Verification items for the finished model (mm, model axes). A direction names the side the tool comes from. Round coordinates to 2 decimals unless told otherwise and drop trailing zeros. Loops run counter-clockwise (first coordinate to the right, second up) from the corner with the lowest first, then second, coordinate; pieces in that order, holes last. Notation, with made-up numbers: M 32,86 L 73,86 A31 cw 73,122 Z; hole C 75,-25.75 d2. An arc over 180 degrees is marked long. Write item = value, one per line. Start each with the question number.
Autodesk Fusion 360 part; units mm, degrees
sketch "Sketch1" plane through (0, 0, 0) normal (0, 1, 0) x (1, 0, 0)
  line L0 (28.15, 28.15) -> (-28.15, 28.15)
  line L1 (-28.15, 28.15) -> (-28.15, -28.15)
  line L2 (-28.15, -28.15) -> (28.15, -28.15)
  line L3 (28.15, -28.15) -> (28.15, 28.15)
  line L4 (28.15, 28.15) -> (-28.15, -28.15) construction
  line L5 (-28.15, 28.15) -> (28.15, -28.15) construction
  line L6 (28.15, 28.15) -> (23.85, 28.15)
  line L7 (23.85, 28.15) -> (23.85, 23.85)
  circle A0 centre (23.85, 23.85) radius 2.5
  circle A1 centre (-23.85, 23.85) radius 2.5
  circle A2 centre (-23.85, -23.85) radius 2.5
  circle A3 centre (23.85, -23.85) radius 2.5
  line L8 (32, 32) -> (-32, 32)
  line L9 (-32, 32) -> (-32, -32)
  line L10 (-32, -32) -> (32, -32)
  line L11 (32, -32) -> (32, 32)
  line L12 (32, 32) -> (-32, -32) construction
  line L13 (-32, 32) -> (32, -32) construction
  circle A4 centre (0, 0) radius 19.25
  dimension "d1" = 56.3
  dimension "d2" = 56.3
  dimension "d3" = 4.3
  dimension "d4" = 4.3
  dimension "d5" = 5
  dimension "d7" = 360
  dimension "d8" = 64
  dimension "d9" = 38.5
extrude "Extrude1" add sketch "Sketch1" along normal blind 4 contours L0 L1 L2 L3 L6 | L8 L9 L10 L11
sketch "Sketch2" plane through (0, 0, 0) normal (0, 1, 0) x (1, 0, 0)
  circle A0 centre (-23.85, 23.85) radius 2.5
  circle A1 centre (23.85, 23.85) radius 2.5
  circle A2 centre (0, 0) radius 19.25
  circle A3 centre (23.85, -23.85) radius 2.5
  circle A4 centre (-23.85, -23.85) radius 2.5
  line L0 (32, 32) -> (32, -32)
  line L1 (32, -32) -> (-32, -32)
  line L2 (-32, -32) -> (-32, 32)
  line L3 (-32, 32) -> (32, 32)
  line L4 (-28.15, 28.15) -> (-28.15, -28.15)
  line L5 (-32, 32) -> (-32, -32)
  line L6 (-28.15, -28.15) -> (-32, -28.15)
  line L7 (-28.15, 28.15) -> (-32, 28.15)
extrude "Extrude2" add sketch "Sketch2" against normal blind 54.2 contours L2 L4 L5 L6 L7
sketch "Sketch3" plane through (-32, 0, 0) normal (-1, 0, 0) x (0, 0, 1)
  line L0 (-32, 0) -> (-28.15, 0)
  line L1 (-28.15, 0) -> (-28.15, -54.2)
  line L2 (-28.15, -54.2) -> (28.15, -54.2)
  line L3 (28.15, -54.2) -> (28.15, 0)
  line L4 (28.15, 0) -> (32, 0)
  line L5 (32, 0) -> (32, 4)
  line L6 (32, 4) -> (-32, 4)
  line L7 (-32, 4) -> (-32, 0)
  line L8 (0, -54.2) -> (10, -54.2)
  line L9 (10, -54.2) -> (-10, -54.2)
  line L10 (-10, -54.2) -> (-10, -49.2)
  line L11 (-10, -49.2) -> (10, -49.2)
  line L12 (10, -49.2) -> (10, -54.2)
  dimension "d14" = 10
  dimension "d15" = 20
  dimension "d16" = 5
extrude "Extrude3" add sketch "Sketch3" along normal blind 15 contours L2 L8 L9 L10 L11 L12
sketch "Sketch4" plane through (0, -49.2, 0) normal (0, 1, 0) x (-1, 0, 0)
  line L0 (32, 10) -> (32, -10)
  line L1 (32, -10) -> (47, -10)
  line L2 (47, -10) -> (47, 10)
  line L3 (47, 10) -> (32, 10)
  line L4 (32, 0) -> (39, 0)
  circle A0 centre (39, 0) radius 2.75
  dimension "d19" = 7
  dimension "d20" = 5.5
extrude "Extrude4" cut sketch "Sketch4" against normal blind 19 contours A0
extrude "Extrude7" cut sketch "Sketch1" along normal blind 5 contours L8 L9 L10 L11
sketch "Sketch7" plane through (0, 0, 0) normal (0, 1, 0) x (1, 0, 0)
  line L0 (-28.15, 28.15) -> (-28.15, -28.15)
  line L1 (-28.15, -28.15) -> (28.15, -28.15)
  line L2 (28.15, -28.15) -> (28.15, 28.15)
  line L3 (28.15, 28.15) -> (-28.15, 28.15)
  circle A0 centre (-23.85, 23.85) radius 2.5
  circle A1 centre (23.85, 23.85) radius 2.5
  circle A2 centre (0, 0) radius 19.25
  circle A3 centre (23.85, -23.85) radius 2.5
  circle A4 centre (-23.85, -23.85) radius 2.5
  line L4 (-28.15, -28.15) -> (-32, -28.15)
  line L5 (-28.15, 28.15) -> (-32, 28.15)
  line L6 (-32, 28.15) -> (-32, -28.15)
  line L7 (-28.15, -28.15) -> (-28.15, 28.15)
extrude "Extrude8" add sketch "Sketch7" along normal blind 4 contours L0 L4 L5 L6 L7
sketch "Sketch8" plane through (-28.15, 0, 0) normal (1, 0, 0) x (0, 0, -1)
  line L0 (28.15, 0) -> (-28.15, 0)
  line L1 (-28.15, 0) -> (-28.15, -54.2)
  line L2 (-28.15, -54.2) -> (28.15, -54.2)
  line L3 (28.15, -54.2) -> (28.15, 0)
  line L4 (-28.15, -54.2) -> (-18.15, -54.2)
  line L5 (-18.15, -54.2) -> (-28.15, -54.2)
  line L6 (-28.15, -54.2) -> (-28.15, 0)
  line L7 (-28.15, 0) -> (-18.15, 0)
  line L8 (-18.15, 0) -> (-18.15, -54.2)
  line L9 (28.15, -54.2) -> (18.15, -54.2)
  line L10 (18.15, -54.2) -> (28.15, -54.2)
  line L11 (28.15, -54.2) -> (28.15, 0)
  line L12 (28.15, 0) -> (18.15, 0)
  line L13 (18.15, 0) -> (18.15, -54.2)
  dimension "d36" = 10
  dimension "d37" = 10
extrude "Extrude9" cut sketch "Sketch8" against normal blind 4 contours L0 L2 L3 L9 L10 L11 L12 L13 | L0 L1 L2 L4 L5 L6 L7 L8
sketch "Sketch9" plane through (0, 4, 0) normal (0, 1, 0) x (-1, 0, 0)
  line L0 (32, 28.15) -> (-28.15, 28.15)
  line L1 (-28.15, 28.15) -> (-28.15, -28.15)
  line L2 (-28.15, -28.15) -> (32, -28.15)
  line L3 (32, -28.15) -> (32, 28.15)
  circle A0 centre (23.85, -23.85) radius 2.5
  circle A1 centre (-23.85, -23.85) radius 2.5
  circle A2 centre (0, 0) radius 19.25
  circle A3 centre (-23.85, 23.85) radius 2.5
  circle A4 centre (23.85, 23.85) radius 2.5
  line L4 (-28.15, 0) -> (-28.15, -10)
  line L5 (-28.15, -10) -> (-23.15, -10)
  line L6 (-23.15, -10) -> (-23.15, 10)
  line L7 (-23.15, 10) -> (-28.15, 10)
  line L8 (-28.15, 10) -> (-28.15, -10)
  dimension "d40" = 10
  dimension "d41" = 5
  dimension "d42" = 20
extrude "Extrude10" add sketch "Sketch9" along normal blind 15 contours L1 L4 L5 L6 L7 L8
sketch "Sketch10" plane through (23.15, 0, 0) normal (-1, 0, 0) x (0, 0, 1)
  line L0 (-10, 4) -> (10, 4)
  line L1 (10, 4) -> (10, 19)
  line L2 (10, 19) -> (-10, 19)
  line L3 (-10, 19) -> (-10, 4)
  line L4 (0, 4) -> (0, 11)
  circle A0 centre (0, 11) radius 2.8
  dimension "d45" = 7
  dimension "d46" = 5.6
extrude "Extrude11" cut sketch "Sketch10" against normal blind 13 contours A0
1. Gauge pin test, flat ends, axial feed: P1, Ø17, axis at x = -13, z = 1, coming from the -Y side; P2, Ø10, axis at y = -47, z = -21, coming from the +X side; P3, Ø8, axis at x = 14.5, z = 15, coming from the +Y side; P4, Ø3, axis at x = -23.85, z = 23.85, coming from the -Y side. Record the tip position at first contact, or that the pin passes through.
2. Thickness scan on line 1 (X direction, y = 2.9, z = -23.85); line 2 (Z direction, x = 23.85, y = 3.05); line 3 (X direction, y = -51.8, z = 0). Record the ranges inside material, lowest first.
3. Section check D-D, the plane z = -11. Enter the section's corners in (x, y), and give its area (3 significant figures).
4. Section check A-A, the plane y = 11. Enter the section's corners in (x, z).
5. Section check C-C, the plane x = -23.85. Enter the section's corners in (y, z).
6. Tool access check on faces 4 (the flat face through (-41.1, -49.2, -2.4)), 5 (the flat face through (-30, -27, -18.15)), 6 (the flat face through (-39, -52, 10)). Record the directions out of +Z, -Z, +X, -X, +Y, -Y that give a thin tool (end or side, any length) a straight path to the whole face; none if there is none.
7. Mould release check, pull along Z, two halves, no side actions. Record for faces 1 (the flat face through (28.15, 7, 0)), 2 (the cylindrical face through (-36.253, -51.665, 0.121)), 3 (the flat face through (26, 11, 10)): pulls with the +Z half, pulls with the -Z half, needs draft (parallel to the pull), parting line crosses it, or undercut.
8. Section check B-B, the plane z = 23.85. Enter the section's corners in (x, y).
Computed values:
q1.P1 = 0
q1.P2 = -28.15
q1.P3 = 4
q1.P4 = through
q2.line_1 = -32 to -26.35, -21.35 to 21.35, 26.35 to 28.15
q2.line_2 = -28.15 to -26.35, -21.35 to 21.35, 26.35 to 28.15
q2.line_3 = -47 to -41.75, -36.25 to -28.15
q3.outline = M -32,-54.2 L -28.15,-54.2 L -28.15,0 L -15.8,0 L -15.8,4 L -32,4 Z; M 15.8,0 L 28.15,0 L 28.15,4 L 15.8,4 Z
q3.area = 323 mm2
q4.outline = M 23.15,-10 L 28.15,-10 L 28.15,-2.8 L 23.15,-2.8 Z; M 23.15,2.8 L 28.15,2.8 L 28.15,10 L 23.15,10 Z
q5.outline = M 0,-28.15 L 4,-28.15 L 4,-26.35 L 0,-26.35 Z; M 0,-21.35 L 4,-21.35 L 4,21.35 L 0,21.35 Z; M 0,26.35 L 4,26.35 L 4,28.15 L 0,28.15 Z
q6.face_4 = +Z, -Z, -X, +Y
q6.face_5 = -Z, +X, -X, -Y
q6.face_6 = +Z, -X, +Y, -Y
q7.face_1 = needs draft
q7.face_2 = undercut
q7.face_3 = pulls with the +Z half
q8.outline = M -32,0 L -26.35,0 L -26.35,4 L -32,4 Z; M -21.35,0 L 21.35,0 L 21.35,4 L -21.35,4 Z; M 26.35,0 L 28.15,0 L 28.15,4 L 26.35,4 Z
